Read the model definition and answer for the solid it produces. Units are mm, in the model's axes. Face numbers are marked on the shaded views. A direction names the side the tool comes from. Coordinates: 2 decimals unless noted, no trailing zeros. Write each loop counter-clockwise with the first axis right and the second up, starting at its lowest first coordinate (ties: lowest second). Pieces come first, ordered by that corner, then holes. Notation, with made-up numbers: M 89,75.5 L 133,75.5 A29 cw 133,96.5 Z; hole C 9,-18.75 d7. An arc over 180 degrees is marked long. Write item = value, one per line.
Autodesk Inventor part; units mm, degrees
ref_plane "Work Plane1" through (6, 0, 0) normal (1, 0, 0) x (0, 0, -1)
ref_plane "YZ Plane" through (0, 0, 0) normal (1, 0, 0) x (0, 1, 0)
ref_plane "XZ Plane" through (0, 0, 0) normal (0, 1, 0) x (-1, 0, 0)
sketch "Sketch2" plane through (0, 0, 0) normal (1, 0, 0) x (0, 1, 0)
  line L0 (0, 0) -> (15, 0)
  line L1 (15, 0) -> (15, -10)
  line L2 (15, -10) -> (0, -10)
  line L3 (0, -10) -> (0, 0)
  dimension "d4" = 15
  dimension "d5" = 10
extrude "Extrusion2" add sketch "Sketch2" along normal blind 12
sketch "Sketch3" plane through (0, 0, 0) normal (0, 0, 1) x (1, 0, 0)
  line L0 (0, 0) -> (1, 0)
  line L1 (0, 0) -> (12, 0)
  line L2 (1, 0) -> (1, 13.5)
  line L3 (1, 13.5) -> (11, 13.5)
  line L4 (11, 13.5) -> (11, 0)
  line L5 (11, 0) -> (1, 0)
  dimension "d8" = 1
  dimension "d9" = 13.5
  dimension "d10" = 10
extrude "Extrusion3" cut sketch "Sketch3" against normal blind 8
sketch "Sketch4" plane through (0, 0, -10) normal (0, 0, -1) x (-1, 0, 0)
  line L0 (0, 15) -> (-12, 15)
  line L1 (0, 0) -> (-12, 0)
  line L2 (-12, 15) -> (0, 15)
  line L3 (0, 15) -> (0, 0)
  line L4 (0, 0) -> (-12, 0)
  line L5 (-12, 0) -> (-12, 15)
extrude "Extrusion4" add sketch "Sketch4" along normal blind 2
sketch "Sketch5" plane through (0, 0, -8) normal (0, 0, 1) x (1, 0, 0)
  line L0 (1, 13.5) -> (11, 13.5)
  line L1 (6, 13.5) -> (6, 10)
  line L2 (6, 10) -> (6, 3.5)
  circle A0 centre (6, 10) radius 1.2295
  circle A1 centre (6, 3.5) radius 1.2295
  point P0 (0, 0)
  dimension "d15" = 3.5
  dimension "d16" = 6.5
  dimension "d17" = 2.459
  dimension "d18" = 2.459
extrude "Extrusion5" cut sketch "Sketch5" against normal blind 4
sketch "Sketch6" plane through (0, 0, -8) normal (0, 0, 1) x (1, 0, 0)
  circle A0 centre (6, 10) radius 1.2295
  circle A1 centre (6, 10) radius 2.7
  circle A2 centre (6, 3.5) radius 1.2295
  circle A3 centre (6, 3.5) radius 2.7
  point P0 (0, 0)
  dimension "d21" = 5.4
  dimension "d22" = 5.4
extrude "Extrusion6" cut sketch "Sketch6" against normal blind 1.1
sketch "Sketch15" plane through (12, 0, 0) normal (1, 0, 0) x (0, 0, -1)
  line L0 (0, 15) -> (12, 15)
  line L1 (12, 15) -> (12, 0)
  line L2 (0, 15) -> (12, 15)
  line L3 (12, 15) -> (12, 0)
  line L4 (12, 0) -> (0, 0)
  line L5 (0, 0) -> (0, 15)
extrude "Extrusion14" add sketch "Sketch15" along normal blind 4
ref_plane "Work Plane1" through (6, 0, 0) normal (1, 0, 0) x (0, 0, -1)
mirror "Mirror1" about plane through (6, 0, 0) normal (1, 0, 0) of "Extrusion14"
sketch "Sketch16" plane through (1, 0, -8) normal (0, -1, 0) x (1, 0, 0)
  line L0 (10, 0) -> (0, 0)
  line L1 (5, 0) -> (7.5, 0)
  line L2 (7.5, 0) -> (7.5, -4)
  line L3 (-5, -4) -> (15, -4)
  line L4 (7.5, -4) -> (2.5, -4)
  line L5 (2.5, -4) -> (2.5, 0)
  line L6 (2.5, 0) -> (5, 0)
  point P0 (-1, 8)
  dimension "d61" = 2.5
  dimension "d62" = 4
  dimension "d63" = 5
  dimension "d64" = 4
extrude "Extrusion15" add sketch "Sketch16" along normal blind 10
sketch "Sketch18" plane through (0, 0, -12) normal (0, 0, -1) x (-1, 0, 0)
  line L0 (-16, 15) -> (4, 15)
  line L1 (4, 0) -> (-3.5, 0)
  line L2 (-16, 15) -> (4, 15)
  line L3 (4, 15) -> (4, 0)
  line L4 (4, 0) -> (-16, 0)
  line L5 (-16, 0) -> (-16, 15)
  line L6 (-8.5, -10) -> (-3.5, -10)
  line L7 (-3.5, 0) -> (-8.5, 0)
  line L8 (-8.5, 0) -> (-8.5, -10)
  line L9 (-8.5, -10) -> (-3.5, -10)
  line L10 (-3.5, -10) -> (-3.5, 0)
  circle A0 centre (-6, 3.5) radius 1.2295
  circle A1 centre (-6, 3.5) radius 1.2295
  circle A2 centre (-6, 10) radius 1.2295
  circle A3 centre (-6, 10) radius 1.2295
  point P0 (0, 0)
extrude "Extrusion16" add sketch "Sketch18" along normal blind 1
sketch "Sketch19" plane through (16, 0, 0) normal (1, 0, 0) x (0, 0, -1)
  line L0 (0, 15) -> (13, 15)
  line L1 (0, 15) -> (0, 40)
  line L2 (-5, 45) -> (-12, 45)
  line L3 (13, 45) -> (13, 15)
  arc A0 (0, 40) -> (-5, 45) centre (-5, 40) ccw
  line L4 (-12, 67) -> (0, 67)
  line L5 (0, 67) -> (13, 56)
  line L6 (13, 56) -> (13, 45)
  line L7 (-8, 56) -> (-12, 67)
  line L8 (-8, 56) -> (-12, 45)
  point P0 (0, 0)
  point P1 (0, 45)
  dimension "d69" = 30
  dimension "d76" = 22
extrude "Extrusion17" add sketch "Sketch19" against normal blind 20
properties part number "20mm_x_20mm"
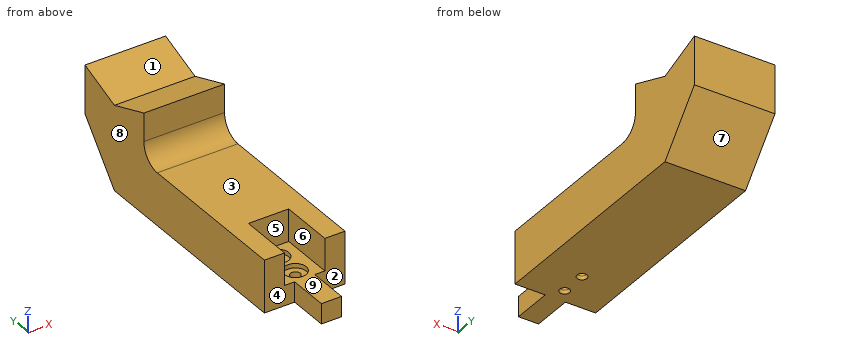
Item 1: Find section B-B (x = 12.5). Determine the outline of the cut face in (y, z).
Worked answers:
outline = M 0,-13 L 56,-13 L 67,0 L 67,12 L 56,8 L 45,12 L 45,5 A5 cw 40,0 L 0,0 Z
Item 2: Find section D-D (y = 35). Determine the outline of the cut face in (x, z).
Worked answers:
outline = M -4,-13 L 16,-13 L 16,0 L -4,0 Z
Item 3: For a pull along X with two mould halves and no side action, classify the marked faces 6, 7, 8 and 9 as released by +X, released by -X, zero draft, split by the parting line, or undercut.
Worked answers:
face_6 = undercut
face_7 = zero draft
face_8 = released by -X
face_9 = undercut
Item 4: Find section A-A (y = 10). Determine the outline of the cut face in (x, z), and give its area (3 significant figures).
Worked answers:
outline = M -4,-13 L 4.77,-13 L 4.77,-9.1 L 3.3,-9.1 L 3.3,-8 L 1,-8 L 1,0 L -4,0 Z; M 7.23,-13 L 16,-13 L 16,0 L 11,0 L 11,-8 L 8.7,-8 L 8.7,-9.1 L 7.23,-9.1 Z
area = 164 mm²
Item 5: Flat-ended cylindrical pins translate along their axes: pin 1 (2 mm diameter, centred on x = 6, y = 10, fed in from +Z); pin 2 (3 mm diameter, centred on x = 6, y = 3.5, fed in from +Z); pin 3 (12 mm diameter, centred on x = 12.5, z = 1.5, fed in from -Y); pin 4 (7.5 mm diameter, centred on x = 7.5, z = 9.5, fed in from -Y). Find the tip coordinate at first contact, or state that the pin passes through.
Worked answers:
pin_1 = through
pin_2 = -9.1
pin_3 = 0
pin_4 = 45
Item 6: Which of the six approach directions +Z, -Z, +X, -X, +Y, -Y give full straight-line access (tool end or side, diameter ignored) to the marked faces 1, 2, 3, 4 and 5?
Worked answers:
face_1 = +Z, +X, -X
face_2 = +Z, -Z, +X, -Y
face_3 = +Z, +X, -X, -Y
face_4 = +Z, -Z, -X, -Y
face_5 = +Z, -Y
Item 7: Consider line 1 along X through (y, z) = (10, -12.25); line 2 along Y through (x, z) = (6, -12.6); line 3 along Y through (x, z) = (6, -10.75). Determine where each line is inside the solid, lowest interval first. Write a range as from..to.
Worked answers:
line_1 = -4..4.77, 7.23..16
line_2 = -10..2.27, 4.73..8.77, 11.23..56.34
line_3 = -10..2.27, 4.73..8.77, 11.23..57.9
Item 8: Find section C-C (x = 6.5). Determine the outline of the cut face in (y, z), and give its area (3 significant figures).
Worked answers:
outline = M -10,-13 L 2.38,-13 L 2.38,-9.1 L 0.85,-9.1 L 0.85,-8 L -10,-8 Z; M 4.62,-13 L 8.88,-13 L 8.88,-9.1 L 7.35,-9.1 L 7.35,-8 L 6.15,-8 L 6.15,-9.1 L 4.62,-9.1 Z; M 11.12,-13 L 56,-13 L 67,0 L 67,12 L 56,8 L 45,12 L 45,5 A5 cw 40,0 L 13.5,0 L 13.5,-8 L 12.65,-8 L 12.65,-9.1 L 11.12,-9.1 Z
area = 938 mm²
